Source: three-view drawing plus pictorial views. Frame: mm from the lowest corner of the part. A direction names the side the tool comes from. Give positions to 0.01 mm unless a question says otherwise; leave off trailing zeros. Order: outer loops, then holes, each group sorted by start corner. A loop starts at its lowest first (then second) coordinate and runs counter-clockwise, first axis right, second up. Notation, with made-up numbers: (89.5, -33) -> (93.5, -33) arc R28 cw to (93.5, -8) -> close; hole circle Ø7 at (28, 28). An arc over 180 degrees is marked (long way). Answer in a Markdown table with one row per item. Add a question column.
Q1. Cut plane B-B on x = 4. Return the cut outline in (y, z), and give its area (3 significant figures).
Q2. Set-up query: the marked faces 5 and 6. Return all of +Z, -Z, +X, -X, +Y, -Y with unobstructed straight access to the full face (end or side cutting, diameter ignored); none if empty.
Q3. Pull-direction query (X, two-part tool) for the marked faces 1, 2, 3 and 4; classes: +X half, -X half, draft (parallel to the pull), parting line (faces both ways), or undercut.
Q4. Contact query for flat-ended pins moving along their axis: P1, Ø1.5, axis at x = 1, y = 2.5, coming from the -Z side; P2, Ø4, axis at x = 4, z = 4.25, coming from the -Y side; P3, Ø1, axis at y = 3, z = 3, coming from the +X side; P4, Ø1.8, axis at x = 4.5, z = 4.5, coming from the -Y side. Output: stop coordinate, or through.
Q5. Cut plane D-D on z = 6.25. Return the cut outline in (x, y) (1 decimal).
Q6. Line query: line 1 along Z through (x, y) = (2.75, 2.1) (1 decimal); line 2 along Y through (x, z) = (6.5, 4.5); line 3 along Y through (x, z) = (5, 5.5). Output: solid intervals per line, ascending. Write a range as from..to.
Q7. Cut plane C-C on y = 2.8. Return the cut outline in (x, z).
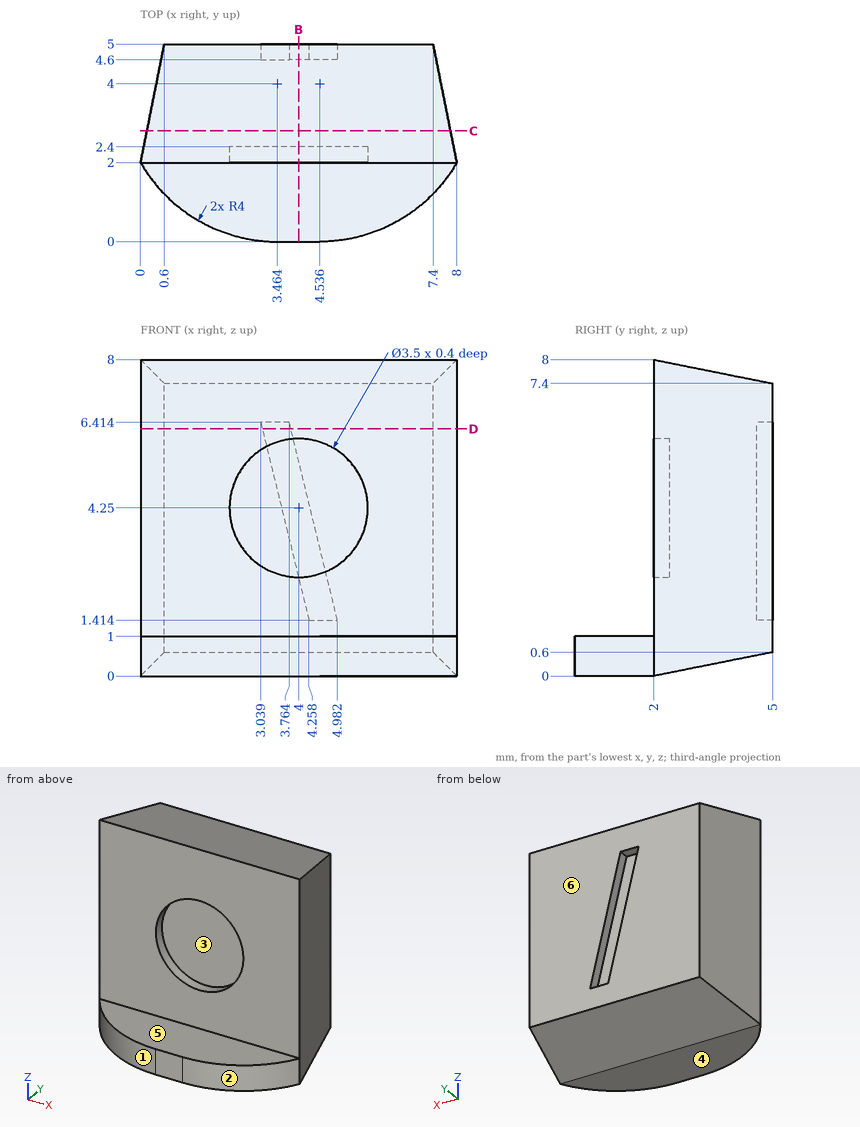
Completed:
| question | item | result |
|---|---|---|
| 1 | outline | (0, 0) -> (2, 0) -> (5, 0.6) -> (5, 2.47) -> (4.6, 2.47) -> (4.6, 5.45) -> (5, 5.45) -> (5, 7.4) -> (2, 8) -> (2, 6) -> (2.4, 6) -> (2.4, 2.5) -> (2, 2.5) -> (2, 1) -> (0, 1) -> close |
| 1 | area | 21.6 mm² |
| 2 | face 5 | +Z, +X, -X, -Y |
| 2 | face 6 | +Z, -Z, +X, -X, +Y |
| 3 | face 1 | -X half |
| 3 | face 2 | +X half |
| 3 | face 3 | undercut |
| 3 | face 4 | draft |
| 4 | P1 | stops at z = 0 |
| 4 | P2 | stops at y = 2 |
| 4 | P3 | stops at x = 7.9 |
| 4 | P4 | stops at y = 2.4 |
| 5 | outline | (0, 2) -> (8, 2) -> (7.4, 5) -> (3.8, 5) -> (3.8, 4.6) -> (3.1, 4.6) -> (3.1, 5) -> (0.6, 5) -> close |
| 6 | line 1 | z = 0..3, 5.5..8 |
| 6 | line 2 | y = 2..5 |
| 6 | line 3 | y = 2.4..5 |
| 7 | outline | (0.16, 0.16) -> (7.84, 0.16) -> (7.84, 7.84) -> (0.16, 7.84) -> close |
